Build history of the part. All positions in model axes, mm. Coordinates: 2 decimals unless noted, no trailing zeros. Loops run counter-clockwise (first coordinate to the right, second up) from the corner with the lowest first, then second, coordinate; pieces in that order, holes last.
(1) Slice it at D-D (x = -134.5). Give the cut face in (y, z), and give its area (3 significant figures).
(2) Slice it at B-B (x = 155.5). Give the cut face in (y, z), and give its area (3 significant figures).
(3) Slice it at A-A (y = -20). Give the cut face in (x, z), and give its area (3 significant figures).
(4) Slice it at C-C (z = 1.25). Give the number of separate pieces and of enclosed holes in the cut face, and give its area (3 significant figures).
(5) Wall check: L1, parallel to Y at x = 2.5, z = 2.05; L2, parallel to Y at x = -88.5, z = 1.8; L3, parallel to X at y = 106.5, z = 0.95. Give the ranges that are in metal, low to high.
(6) Flat gauge pin, fed straight in: P1, Ø2, axis at y = 121, z = 1.5, coming from the +X side. Where does the tip first touch, or does it go through?
Solid Edge part; units mm, degrees
sketch "Sketch1" plane through (0, 0, 0) normal (0, 0, 1) x (1, 0, 0)
  line L0 (-200, -115) -> (200, -115)
  line L1 (200, -115) -> (200, 115)
  line L2 (200, 115) -> (-200, 115)
  line L3 (-200, 115) -> (-200, -115)
  line L4 (-160, 115) -> (-160, 125)
  line L5 (-160, 125) -> (-200, 125)
  line L6 (-200, 125) -> (-200, 115)
  line L7 (-200, 115) -> (-160, 115)
  line L8 (-120, 115) -> (-80, 115)
  line L9 (-80, 115) -> (-80, 125)
  line L10 (-80, 125) -> (-120, 125)
  line L11 (-120, 125) -> (-120, 115)
  line L12 (-40, 115) -> (0, 115)
  line L13 (0, 115) -> (0, 125)
  line L14 (0, 125) -> (-40, 125)
  line L15 (-40, 125) -> (-40, 115)
  line L16 (40, 115) -> (80, 115)
  line L17 (80, 115) -> (80, 125)
  line L18 (80, 125) -> (40, 125)
  line L19 (40, 125) -> (40, 115)
  line L20 (120, 115) -> (160, 115)
  line L21 (160, 115) -> (160, 125)
  line L22 (160, 125) -> (120, 125)
  line L23 (120, 125) -> (120, 115)
  line L24 (-150, -106) -> (-170, -106)
  line L25 (-170, -106) -> (-170, -110)
  line L26 (-170, -110) -> (-150, -110)
  line L27 (-150, -110) -> (-150, -106)
  line L28 (-90, -110) -> (-70, -110)
  line L29 (-70, -110) -> (-70, -106)
  line L30 (-70, -106) -> (-90, -106)
  line L31 (-90, -106) -> (-90, -110)
  line L32 (-10, -110) -> (10, -110)
  line L33 (10, -110) -> (10, -106)
  line L34 (10, -106) -> (-10, -106)
  line L35 (-10, -106) -> (-10, -110)
  line L36 (70, -110) -> (90, -110)
  line L37 (90, -110) -> (90, -106)
  line L38 (90, -106) -> (70, -106)
  line L39 (70, -106) -> (70, -110)
  line L40 (150, -110) -> (170, -110)
  line L41 (170, -110) -> (170, -106)
  line L42 (170, -106) -> (150, -106)
  line L43 (150, -106) -> (150, -110)
  line L44 (-191, -89) -> (-191, -69)
  line L45 (-191, -69) -> (-195, -69)
  line L46 (-195, -69) -> (-195, -89)
  line L47 (-195, -89) -> (-191, -89)
  line L48 (-191, -29) -> (-191, -9)
  line L49 (-191, -9) -> (-195, -9)
  line L50 (-195, -9) -> (-195, -29)
  line L51 (-195, -29) -> (-191, -29)
  line L52 (-191, 90) -> (-191, 110)
  line L53 (-191, 110) -> (-195, 110)
  line L54 (-195, 110) -> (-195, 90)
  line L55 (-195, 90) -> (-191, 90)
  line L56 (191, -69) -> (191, -89)
  line L57 (191, -89) -> (195, -89)
  line L58 (195, -89) -> (195, -69)
  line L59 (195, -69) -> (191, -69)
  line L60 (195, -29) -> (195, -9)
  line L61 (195, -9) -> (191, -9)
  line L62 (191, -9) -> (191, -29)
  line L63 (191, -29) -> (195, -29)
  line L64 (191, 110) -> (191, 90)
  line L65 (191, 90) -> (195, 90)
  line L66 (195, 90) -> (195, 110)
  line L67 (195, 110) -> (191, 110)
extrude "Protrusion1" add sketch "Sketch1" along normal blind 4
Response values:
1. outline: (-115, 0) - (115, 0) - (115, 4) - (-115, 4) - close
1. area: 920 mm2
2. outline: (-115, 0) - (-110, 0) - (-110, 4) - (-115, 4) - close; (-106, 0) - (125, 0) - (125, 4) - (-106, 4) - close
2. area: 944 mm2
3. outline: (-200, 0) - (-195, 0) - (-195, 4) - (-200, 4) - close; (-191, 0) - (191, 0) - (191, 4) - (-191, 4) - close; (195, 0) - (200, 0) - (200, 4) - (195, 4) - close
3. area: 1,570 mm2
4. separate pieces: 1
4. enclosed holes: 11
4. area: 93,100 mm2
5. L1: y = -115 to -110, -106 to 115
5. L2: y = -115 to -110, -106 to 125
5. L3: x = -200 to -195, -191 to 191, 195 to 200
6. P1: stops at x = 160
